Part print with two shaded views. Sizes in mm from the minimum x, y, z corner. A direction names the side the tool comes from. Coordinates: 2 decimals unless noted, no trailing zeros. Order: outer loops, then holes, each group sorted by start corner. A loop starts at its lowest first (then second) coordinate and runs counter-clockwise, first axis right, second up. Notation, with made-up numbers: (2.5, -1) - (38.5, -1) arc R11 cw to (38.5, 19) - close; hole circle Ø11 at (8, 82). An arc over 180 degrees is marked (long way). Return JSON: item names as keys, results as strings.
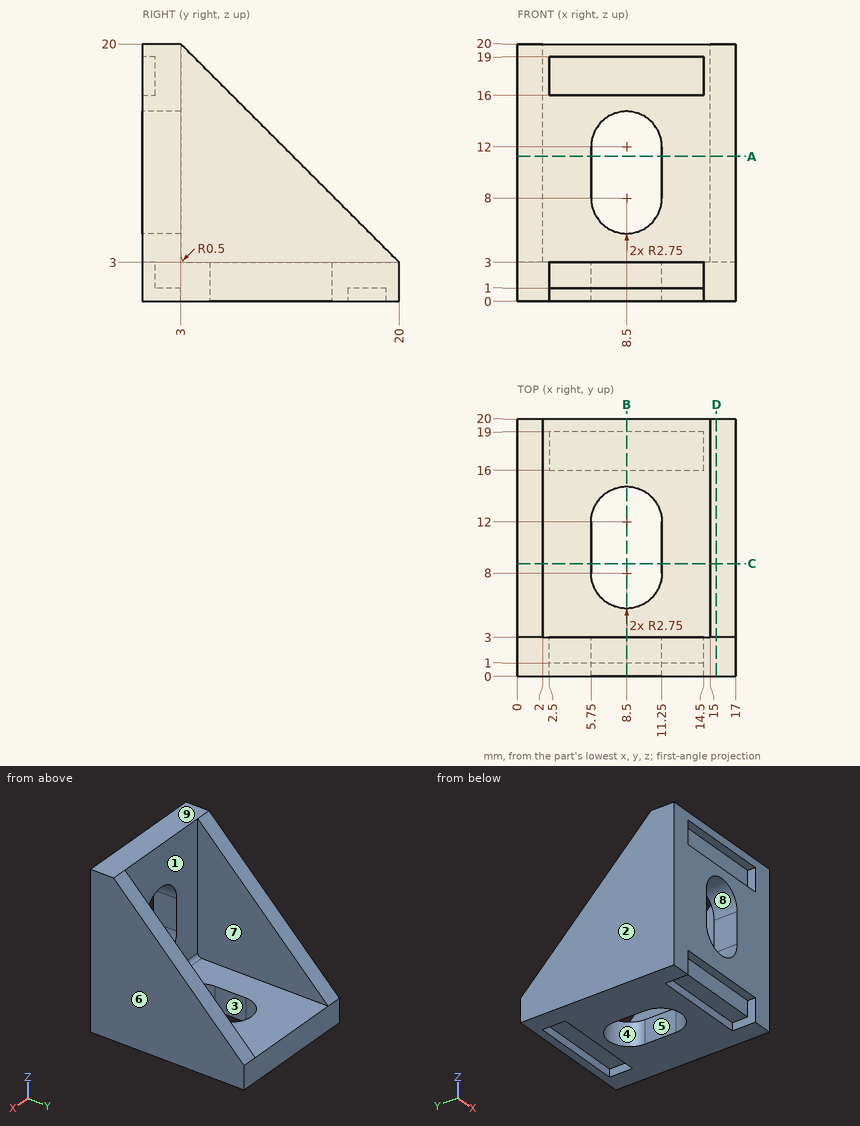
Item 1: Wall check: L1, parallel to X at y = 6.75, z = 12.25; L2, parallel to Y at x = 11.5, z = 11.5. Give the ranges that are in metal, low to high. Write a range as [from, to].
Findings below:
{"L1": "x = [0, 2], [15, 17]", "L2": "y = [0, 3]"}
Item 2: Drop flat-ended pins along their axis: P1, Ø1.1, axis at x = 6, y = 0.5, coming from the -Z side; P2, Ø0.8, axis at x = 6.5, z = 0.5, coming from the -Y side; P3, Ø6.5, axis at x = 10.5, z = 9.5, coming from the +Y side. Give the stop position or say it passes through.
Findings below:
{"P1": "stops at z = 1", "P2": "stops at y = 3", "P3": "stops at y = 3"}
Item 3: Band-saw the part on C-C, the plane y = 8.75. List the corners of the cut face in (x, z), then the cut area to 3 significant figures.
Findings below:
{"outline": "(0, 0) - (5.75, 0) - (5.75, 3) - (2, 3) - (2, 14.25) - (0, 14.25) - close; (11.25, 0) - (17, 0) - (17, 14.25) - (15, 14.25) - (15, 3) - (11.25, 3) - close", "area": "79.5 mm²"}
Item 4: Which spindle directions (+Z, -Z, +X, -X, +Y, -Y) get a long thin tool onto all of the face, cutting with end or side? Do the marked faces 5, 6, 7, 8 and 9. Say none if no direction does.
Findings below:
{"face 5": "+Z, -Z", "face 6": "+Z, -Z, +X, +Y, -Y", "face 7": "+Z, +Y", "face 8": "+Y, -Y", "face 9": "+Z, +X, -X, +Y, -Y"}
Item 5: Mould opens along Y. For the marked faces 1, 2, 3 and 4 say: released by +Y, released by -Y, zero draft, split by the parting line, or undercut.
Findings below:
{"face 1": "released by +Y", "face 2": "zero draft", "face 3": "undercut", "face 4": "undercut"}
Item 6: Band-saw the part on B-B, the plane x = 8.5. List the corners of the cut face in (y, z).
Findings below:
{"outline": "(0, 3) - (1, 3) - (1, 1) - (3, 1) - (3, 0) - (5.25, 0) - (5.25, 3) - (3.5, 3) arc R0.5 cw to (3, 3.5) - (3, 5.25) - (0, 5.25) - close; (0, 14.75) - (3, 14.75) - (3, 20) - (0, 20) - (0, 19) - (1, 19) - (1, 16) - (0, 16) - close; (14.75, 0) - (16, 0) - (16, 1) - (19, 1) - (19, 0) - (20, 0) - (20, 3) - (14.75, 3) - close"}
Item 7: Band-saw the part on A-A, the plane z = 11.25. List the corners of the cut face in (x, y).
Findings below:
{"outline": "(0, 0) - (5.75, 0) - (5.75, 3) - (2, 3) - (2, 11.75) - (0, 11.75) - close; (11.25, 0) - (17, 0) - (17, 11.75) - (15, 11.75) - (15, 3) - (11.25, 3) - close"}
Item 8: Band-saw the part on D-D, the plane x = 15.5. List the corners of the cut face in (y, z), then the cut area to 4 significant figures.
Findings below:
{"outline": "(0, 0) - (20, 0) - (20, 3) - (3, 20) - (0, 20) - close", "area": "255.5 mm²"}
